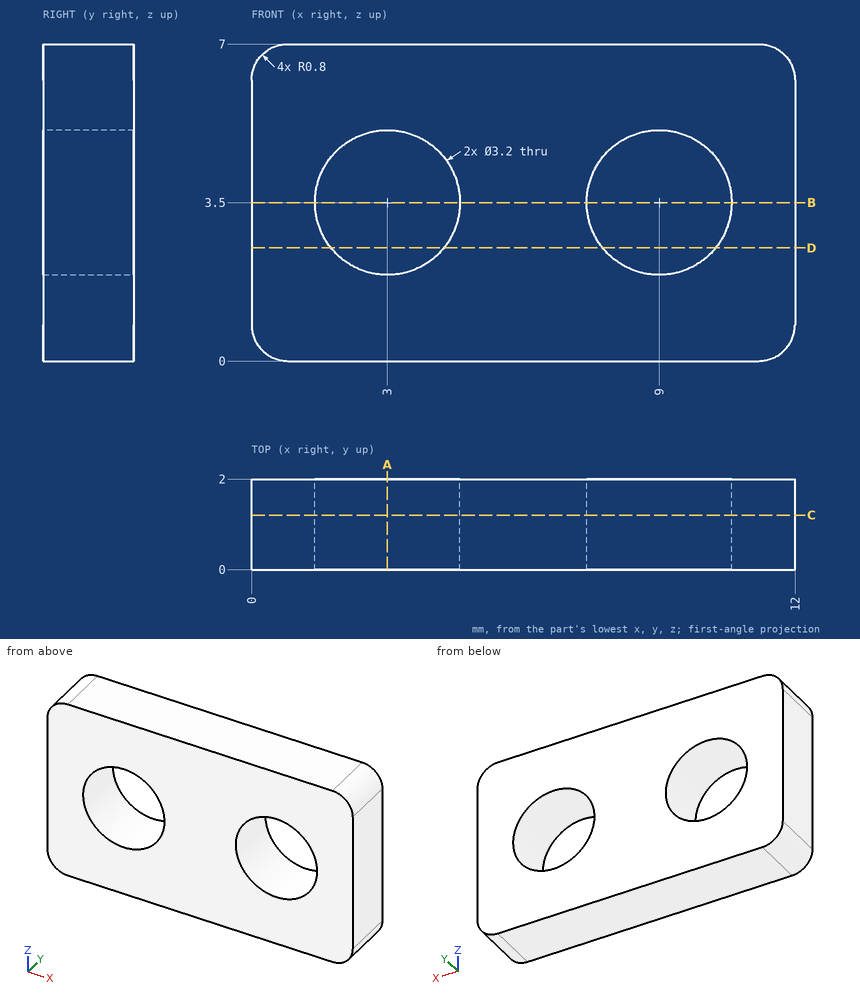
Geometry check sheet. Reference: drawing and pictorial views, mm from the part's lowest x, y, z. Coordinates: 2 decimals unless noted, no trailing zeros. Loops run counter-clockwise (first coordinate to the right, second up) from the corner with the lowest first, then second, coordinate; pieces in that order, holes last. Notation, with made-up numbers: (71, -8.75) -> (114, -8.75) arc R36 ccw to (114, 30.25) -> close; hole circle Ø5 at (71.25, -28). An arc over 180 degrees is marked (long way). Write item = value, one per line. Start each with the question number.
1. Depth check by flat-ended pin: P1, Ø1.9, axis at x = 3, z = 3.5, coming from the -Y side. Enter the tip coordinate at first touch or a pass-through.
2. Material ranges on line 1 (X direction, y = 1.4, z = 3.5); line 2 (X direction, y = 0.9, z = 2.25); line 3 (Z direction, x = 9.25, y = 1.45), recorded low to high.
3. Section check A-A on x = 3. Record the cut outline in (y, z).
4. Section check B-B on z = 3.5. Record the cut outline in (x, y).
5. Section check C-C on y = 1.2. Record the cut outline in (x, z).
6. Section check D-D on z = 2.5. Record the cut outline in (x, y).
Responses:
q1.P1 = through
q2.line_1 = 0 to 1.4, 4.6 to 7.4, 10.6 to 12
q2.line_2 = 0 to 2, 4 to 8, 10 to 12
q2.line_3 = 0 to 1.92, 5.08 to 7
q3.outline = (0, 0) -> (2, 0) -> (2, 1.9) -> (0, 1.9) -> close; (0, 5.1) -> (2, 5.1) -> (2, 7) -> (0, 7) -> close
q4.outline = (0, 0) -> (1.4, 0) -> (1.4, 2) -> (0, 2) -> close; (4.6, 0) -> (7.4, 0) -> (7.4, 2) -> (4.6, 2) -> close; (10.6, 0) -> (12, 0) -> (12, 2) -> (10.6, 2) -> close
q5.outline = (0, 0.8) arc R0.8 ccw to (0.8, 0) -> (11.2, 0) arc R0.8 ccw to (12, 0.8) -> (12, 6.2) arc R0.8 ccw to (11.2, 7) -> (0.8, 7) arc R0.8 ccw to (0, 6.2) -> close; hole circle Ø3.2 at (3, 3.5); hole circle Ø3.2 at (9, 3.5)
q6.outline = (0, 0) -> (1.75, 0) -> (1.75, 2) -> (0, 2) -> close; (4.25, 0) -> (7.75, 0) -> (7.75, 2) -> (4.25, 2) -> close; (10.25, 0) -> (12, 0) -> (12, 2) -> (10.25, 2) -> close
